Input: part model. Units: mm. Frame: model coordinates. Coordinates: 2 decimals unless noted, no trailing zeros. Order: outer loops, then holes, each group sorted by start corner. A loop starts at its lowest first (then second) coordinate and runs counter-clockwise, first axis right, second up. Notation, with made-up numbers: (5, 0) -> (55, 0) arc R24 cw to (55, 12) -> close; hole circle Ø10 at (37.25, -10). An arc over 180 degrees is marked (long way). One line per item, written item: value. Start each with the question number.
Solid Edge part; units mm, degrees
sketch "Sketch1" plane through (0, 0, 0) normal (0, 0, 1) x (1, 0, 0)
  line L0 (0, 12) -> (-10.3923, 6)
  line L1 (-10.3923, 6) -> (-10.3923, -6)
  line L2 (-10.3923, -6) -> (0, -12)
  line L3 (0, -12) -> (10.3923, -6)
  line L4 (10.3923, -6) -> (10.3923, 6)
  line L5 (10.3923, 6) -> (0, 12)
extrude "Protrusion1" add sketch "Sketch1" along normal mid plane 10.8
sketch "Sketch2" plane through (0, 0, 0) normal (0, -1, 0) x (1, 0, 0)
  line L0 (10.3923, -5.4) -> (40.2366, 11.8306)
revolve "RevolvedCutout1" cut sketch "Sketch2" angle 360 about axis through (0, 0, 54) along (0, 0, -1) material side at (25.3394, 0, 3.172)
mirror "Mirror1" about plane through (0, 0, 0) normal (0, 0, 1) of "RevolvedCutout1"
hole "Hole_1" at (0, 0, 5.4) direction (0, 0, -1) diameter 10.106 end through all
properties part number "2"
1) Ray query, line 1 along X through (y, z) = (0, -1.25); line 2 along X through (y, z) = (1.75, 4.5); line 3 along Y through (x, z) = (-4, 5). Return the intervals inside material, ascending. Write a range as from..to.
2) Pin query (flat end, axial travel): pin 1 Ø1.5 at (x, z) = (-6, 2) entering from +Y; pin 2 Ø4 at (x, z) = (-1, -3.5) entering from +Y; pin 3 Ø6 at (y, z) = (9.5, 4) entering from +X; pin 4 Ø6 at (x, z) = (-7, 3) entering from +Y. Return the tip coordinate at first contact, or that it passes through.
3) Mould query, pull axis X, two halves, no side actions, for faces 1 (the conical face through (0.23, -10.67, 5.24)), 2 (the cylindrical face through (-3.075, 4.01, 0.076)), 3 (the flat face through (5.269, 8.958, -0.076)). Classes: +X half, -X half, draft (parallel to the pull), parting line (faces both ways), or undercut.
4) Section query A-A, the plane z = -3. Return the cut outline in (x, y).
Entries:
1. line 1: x = -10.39..-5.05, 5.05..10.39
1. line 2: x = -10.39..-4.74, 4.74..10.39
1. line 3: y = -9.69..-3.09, 3.09..9.69
2. pin 1: stops at y = 8.97
2. pin 2: stops at y = 12
2. pin 3: stops at x = 9.53
2. pin 4: stops at y = 9.69
3. face 1: parting line
3. face 2: undercut
3. face 3: +X half
4. outline: (-10.39, -6) -> (0, -12) -> (10.39, -6) -> (10.39, 6) -> (0, 12) -> (-10.39, 6) -> close; hole circle Ø10.11 at (0, 0)
